Source: CAD feature listing. Evaluate the final solid. Frame: model axes, mm. A direction names the side the tool comes from. Round coordinates to 2 decimals unless told otherwise and drop trailing zeros. Order: outer loops, then holes, each group sorted by start corner. A loop starts at its lowest first (then second) coordinate and runs counter-clockwise, first axis right, second up. Notation, with made-up numbers: (8, 11) - (56, 11) arc R35 ccw to (56, 49) - close; hole circle Ø6 at (-27, 53). An arc over 180 degrees is marked (long way). Put each result on its own line as item: value. Start each with the question number.
1) Section A-A on x = 1.75. Output: boundary loops of the cut face in (y, z), then the cut area to 3 significant figures.
2) Mould query, pull axis Z, two halves, no side actions, for faces 1 (the face through (-8, -2, 28)), 2 (the face through (9.582, -5, 29)), 3 (the face through (-5.418, -5, 15)). Classes: +Z half, -Z half, draft (parallel to the pull), parting line (faces both ways), or undercut.
3) Line query: probe 1 along Z at (x, y) = (-0.25, -5); probe 2 along X at (y, z) = (-3.25, 17.25). Output: solid intervals per line, ascending. Write a range as [from, to].
4) Section D-D on x = -7.75. Output: boundary loops of the cut face in (y, z).
5) Access query for faces 4 (the face through (2, -5, 2)), 5 (the face through (-9, -14.628, 15)), 6 (the face through (-10.915, -1.519, 0.986)), 7 (the face through (-15.418, -5, 15)), 8 (the face through (-10.915, -1.519, 29.014)). Directions: +Z, -Z, +X, -X, +Y, -Y. A direction counts if a zero-diameter tool reaches every point of the face in a straight line with its end or side. Return the directions, or none.
6) Contact query for flat-ended pins moving along their axis: P1, Ø6, axis at y = -4.5, z = 20.5, coming from the +X side; P2, Ø1.5, axis at x = -9.5, y = -2, coming from the -Z side; P3, Ø4.5, axis at x = -8.42, y = -1.63, coming from the +Z side. Output: stop coordinate, or through.
7) Section B-B on y = -6.25. Output: boundary loops of the cut face in (x, z), then the cut area to 3 significant figures.
8) Section C-C on z = 22.25. Output: boundary loops of the cut face in (x, y).
```python
from build123d import *

# Parameters (mm, degrees)
F0_W     = 10
F0_H     = 20
F1_DEPTH = 30
F2_W     = 20
F2_H     = 2
F3_DEPTH = 15
F4_R     = 2.5
F5_DEPTH = 2
F6_R     = 2.5
F7_DEPTH = 2


with BuildPart() as f1:
    # F0 (on Top) → F1 (new body)
    with BuildSketch(Plane.XY):
        with Locations((-10.417764, -4.628471)):
            Rectangle(F0_W, F0_H)
    extrude(amount=F1_DEPTH)

    # F2 (on face) → F3 (join)
    with BuildSketch(Plane.YZ.offset(-5.417764)):
        with Locations((-4.628471, 29)):
            Rectangle(F2_W, F2_H)
        with Locations((-4.628471, 1)):
            Rectangle(F2_W, F2_H)
    extrude(amount=F3_DEPTH)

    # F4 (on Top) → F5 (cut)
    with BuildSketch(Plane.XY):
        with Locations((-8.417764, -1.628471)):
            Circle(F4_R)
    extrude(amount=F5_DEPTH, mode=Mode.SUBTRACT)

    # F6 (on face) → F7 (cut)
    with BuildSketch(Plane.XY.offset(30)):
        with Locations((-8.417764, -1.628471)):
            Circle(F6_R)
    extrude(amount=-F7_DEPTH, mode=Mode.SUBTRACT)


solid = f1.part
```
Answer sheet:
1. outline: (-14.63, 0) - (5.37, 0) - (5.37, 2) - (-14.63, 2) - close; (-14.63, 28) - (5.37, 28) - (5.37, 30) - (-14.63, 30) - close
1. area: 80.0 mm^2
2. face 1: +Z half
2. face 2: draft
2. face 3: undercut
3. probe 1: [0, 2], [28, 30]
3. probe 2: [-15.42, -5.42]
4. outline: (-14.63, 0) - (-4.04, 0) - (-4.04, 2) - (0.78, 2) - (0.78, 0) - (5.37, 0) - (5.37, 30) - (0.78, 30) - (0.78, 28) - (-4.04, 28) - (-4.04, 30) - (-14.63, 30) - close
5. face 4: +X, +Y, -Y
5. face 5: +Z, -Z, +X, -X, -Y
5. face 6: -Z
5. face 7: +Z, -Z, -X, +Y, -Y
5. face 8: +Z
6. P1: x = -5.42
6. P2: z = 2
6. P3: z = 28
7. outline: (-15.42, 0) - (9.58, 0) - (9.58, 2) - (-5.42, 2) - (-5.42, 28) - (9.58, 28) - (9.58, 30) - (-15.42, 30) - close
7. area: 360 mm^2
8. outline: (-15.42, -14.63) - (-5.42, -14.63) - (-5.42, 5.37) - (-15.42, 5.37) - close
